Here's how the part is built. I have some questions about the finished solid (model axes, mm). Round coordinates to 2 decimals unless told otherwise and drop trailing zeros. Write each loop counter-clockwise with the first axis right and the second up, starting at its lowest first coordinate (ties: lowest second). Pieces come first, ordered by that corner, then holes. Notation, with made-up numbers: (-16, -17) - (5, -17) arc R19 cw to (5, -7) - close; hole circle Ø8 at (66.25, 17). An arc over 180 degrees is marked (long way). Use one line per item in the form item = value. Start each with the question number.
1. I want a section at D-D, the plane z = -47. List the corners of the cut face in (x, y) for me.
2. I want a section at A-A, the plane z = -2.5. List the corners of the cut face in (x, y) for me, plus the area to 3 significant figures.
3. I want a section at C-C, the plane y = 2.35. List the corners of the cut face in (x, z) for me, plus the area to 3 significant figures.
4. I want a section at B-B, the plane x = 32. List the corners of the cut face in (y, z) for me, plus the area to 3 significant figures.
5. If I drill on line 1 along X through (y, z) = (1.2, -2.5); line 2 along Z through (x, y) = (21, 1.65); line 3 along X through (y, z) = (1.1, -38), over which ranges is the centre line in solid material (lowest first)?
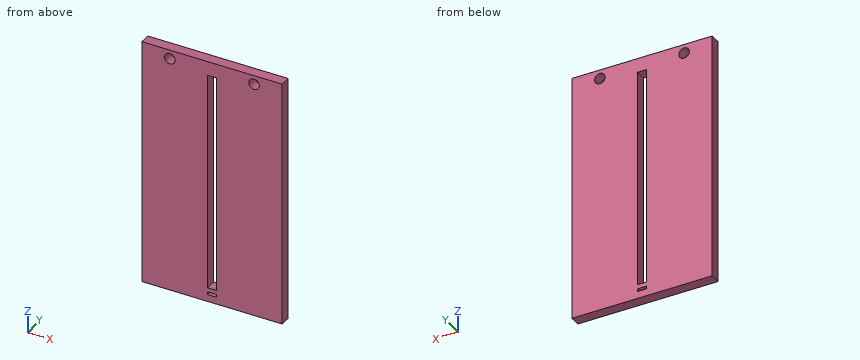
```python
from build123d import *

# Parameters (mm, degrees)
SKETCH1_W           = 40
SKETCH1_H           = 70
BOSS_EXTRUDE1_DEPTH = 3.05
SKETCH4_W           = 2.6
SKETCH4_H           = 62
SKETCH4_H_2         = 0.8
CUT_EXTRUDE1_DEPTH  = 10
SKETCH7_R           = 1.5
CUT_EXTRUDE4_DEPTH  = 10


with BuildPart() as part:
    # Sketch1 → Boss-Extrude1 (new body)
    with BuildSketch(Plane(origin=(0, 0, 0), x_dir=(1, 0, 0), z_dir=(0, 1, 0))):
        with Locations((20, 35)):
            Rectangle(SKETCH1_W, SKETCH1_H)
    extrude(amount=BOSS_EXTRUDE1_DEPTH)

    # Sketch4 → Cut-Extrude1 (cut)
    with BuildSketch(Plane(origin=(0, 3.05, 0), x_dir=(1, 0, 0), z_dir=(0, 1, 0))):
        with Locations((20, 35)):
            Rectangle(SKETCH4_W, SKETCH4_H)
        with Locations((20, 67.6)):
            Rectangle(SKETCH4_W, SKETCH4_H_2)
    extrude(amount=-CUT_EXTRUDE1_DEPTH, mode=Mode.SUBTRACT)

    # Sketch7 → Cut-Extrude4 (cut)
    with BuildSketch(Plane(origin=(0, 3.05, 0), x_dir=(1, 0, 0), z_dir=(0, 1, 0))):
        with Locations(Location((8, 2.5, 0), (0, 0, 270))):
            Circle(SKETCH7_R)
        with Locations(Location((32, 2.5, 0), (0, 0, 270))):
            Circle(SKETCH7_R)
    extrude(amount=-CUT_EXTRUDE4_DEPTH, mode=Mode.SUBTRACT)


solid = part.part
```
Model answer:
q1.outline = (0, 0) - (18.7, 0) - (18.7, 3.05) - (0, 3.05) - close; (21.3, 0) - (40, 0) - (40, 3.05) - (21.3, 3.05) - close
q2.outline = (0, 0) - (6.5, 0) - (6.5, 3.05) - (0, 3.05) - close; (9.5, 0) - (30.5, 0) - (30.5, 3.05) - (9.5, 3.05) - close; (33.5, 0) - (40, 0) - (40, 3.05) - (33.5, 3.05) - close
q2.area = 104 mm2
q3.outline = (0, -70) - (40, -70) - (40, 0) - (0, 0) - close; hole circle Ø3 at (8, -2.5); hole (18.7, -68) - (21.3, -68) - (21.3, -67.2) - (18.7, -67.2) - close; hole (18.7, -66) - (21.3, -66) - (21.3, -4) - (18.7, -4) - close; hole circle Ø3 at (32, -2.5)
q3.area = 2,620 mm2
q4.outline = (0, -70) - (3.05, -70) - (3.05, -4) - (0, -4) - close; (0, -1) - (3.05, -1) - (3.05, 0) - (0, 0) - close
q4.area = 204 mm2
q5.line_1 = 0 to 6.5, 9.5 to 30.5, 33.5 to 40
q5.line_2 = -70 to -68, -67.2 to -66, -4 to 0
q5.line_3 = 0 to 18.7, 21.3 to 40
